Here's how the part is built. I have some questions about the finished solid (model axes, mm). Face numbers are marked on the shaded views. A direction names the side the tool comes from. Coordinates: 2 decimals unless noted, no trailing zeros. Order: outer loops, then holes, each group sorted by start corner. A loop starts at its lowest first (then second) coordinate and runs counter-clockwise, first axis right, second up.
```python
from build123d import *

# Parameters (mm, degrees)
SKETCH_3_W          = 8
SKETCH_3_H          = 16.823898374
CUT_EXTRUDE_1_DEPTH = 10
SKETCH_5_OUTSIDE_W  = 23.858
SKETCH_5_OUTSIDE_H  = 27.858
SKETCH_5_OUTSIDE_R  = 8
CUT_EXTRUDE_2_DEPTH = 10
SKETCH_6_R          = 3
EXTRUDE_1_DEPTH     = 6


with BuildPart() as part:
    # 草图2 → 旋转1 (revolve)
    with BuildSketch(Plane(origin=(0, 0, 0), x_dir=(0, 0, -1), z_dir=(1, 0, 0))):
        Polygon((0, 0), (0, 5), (15, 5), (15, 9), (21, 9), (21, 4), (32, 4), (32, 0), align=None)
    revolve(axis=Axis((0, 0, 0), (0, 0, -1)))

    # 草图3 → 切除-拉伸1 (cut)
    with BuildSketch(Plane.XY.offset(-15)):
        with Locations((-11, -0.026043186)):
            Rectangle(SKETCH_3_W, SKETCH_3_H)
        with Locations((11, -0.026043186)):
            Rectangle(SKETCH_3_W, SKETCH_3_H)
    extrude(amount=-CUT_EXTRUDE_1_DEPTH, mode=Mode.SUBTRACT)

    # 草图5 outside → 切除-拉伸2 (cut)
    with BuildSketch(Plane(origin=(0, 0, -21), x_dir=(-1, 0, 0), z_dir=(0, 0, -1))):
        Rectangle(SKETCH_5_OUTSIDE_W, SKETCH_5_OUTSIDE_H)
        Circle(SKETCH_5_OUTSIDE_R, mode=Mode.SUBTRACT)
    extrude(amount=-CUT_EXTRUDE_2_DEPTH, mode=Mode.SUBTRACT)

    # 草图6 → 凸台-拉伸1 (add)
    with BuildSketch(Plane(origin=(0, 0, -32), x_dir=(-1, 0, 0), z_dir=(0, 0, -1))):
        Circle(SKETCH_6_R)
    extrude(amount=EXTRUDE_1_DEPTH)


solid = part.part
```
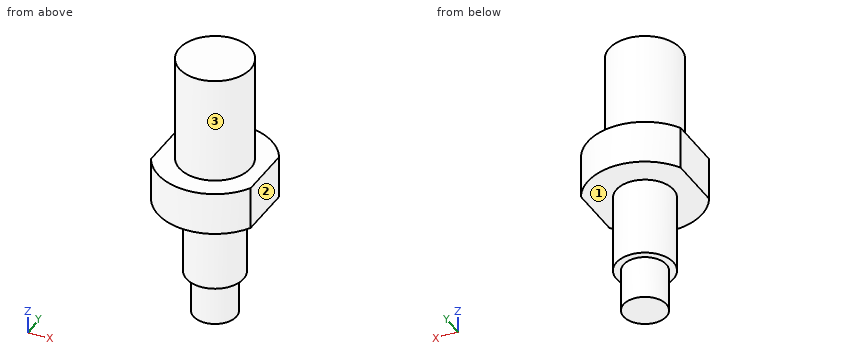
Q1. If we section it at A-A on y = 0: Write out the boundary of the cut face in (x, z), then the cut area to 3 significant figures.
Q2. If we section it at C-C on z = -34: Write out the boundary of the cut face in (x, y).
Q3. If we section it at D-D on x = -3.5: Write out the boundary of the cut face in (y, z).
Q4. For the marked faces 1, 2 and 3, which set-ups out of +Z, -Z, +X, -X, +Y, -Y let a thin tool reach every point of the face, with its end or its side?
Q5. I need wall thicknesses on L1, parallel to Z at x = -3.5, y = -4; L2, parallel to Z at x = -2, y = 4; L3, parallel to Y at x = -3.25, z = -29.5. Which ranges of each line are inside material? Lowest first, please.
Q6. Will these pins go through, and if not, where does the flat tip stop? pin 1 (1 mm diameter, centred on y = -5, z = -31.5, fed in from -X); pin 2 (8 mm diameter, centred on y = -2.5, z = -28, fed in from -X); pin 3 (1 mm diameter, centred on x = 2.5, z = -17, fed in from +Y); pin 4 (4 mm diameter, centred on x = -2.5, z = -26.5, fed in from -Y).
Q7. If we section it at B-B on x = 0: Write out the boundary of the cut face in (y, z), then the cut area to 3 significant figures.
Reply:
1. outline: (-7, -21) - (-4, -21) - (-4, -32) - (-3, -32) - (-3, -38) - (3, -38) - (3, -32) - (4, -32) - (4, -21) - (7, -21) - (7, -15) - (5, -15) - (5, 0) - (-5, 0) - (-5, -15) - (-7, -15) - close
1. area: 358 mm2
2. outline: circle Ø6 at (0, 0)
3. outline: (-7.19, -21) - (-1.94, -21) - (-1.94, -32) - (1.94, -32) - (1.94, -21) - (7.19, -21) - (7.19, -15) - (3.57, -15) - (3.57, 0) - (-3.57, 0) - (-3.57, -15) - (-7.19, -15) - close
4. face 1: -Z
4. face 2: +Z, -Z, +X, +Y, -Y
4. face 3: +Z
5. L1: z = -21 to -15
5. L2: z = -21 to 0
5. L3: y = -2.33 to 2.33
6. pin 1: passes through
6. pin 2: stops at x = -4
6. pin 3: stops at y = 7.75
6. pin 4: stops at y = -3.97
7. outline: (-8, -21) - (-4, -21) - (-4, -32) - (-3, -32) - (-3, -38) - (3, -38) - (3, -32) - (4, -32) - (4, -21) - (8, -21) - (8, -15) - (5, -15) - (5, 0) - (-5, 0) - (-5, -15) - (-8, -15) - close
7. area: 370 mm2
